```python
from build123d import *

# Parameters (mm, degrees)
SKETCH1_R           = 71.12
SKETCH1_R_2         = 12.704134002
SKETCH1_R_3         = 6.35
BOSS_EXTRUDE1_DEPTH = 3.175


with BuildPart() as part:
    # Sketch1 → Boss-Extrude1 (new body, symmetric)
    with BuildSketch(Plane(origin=(0, 0, 0), x_dir=(1, 0, 0), z_dir=(0, 1, 0))):
        Circle(SKETCH1_R)
        with Locations((-25.296602045, 14.605)):
            Circle(SKETCH1_R_2, mode=Mode.SUBTRACT)
        with Locations((-25.296602045, -14.605)):
            Circle(SKETCH1_R_2, mode=Mode.SUBTRACT)
        with Locations((0, -29.21)):
            Circle(SKETCH1_R_2, mode=Mode.SUBTRACT)
        with Locations((25.296602045, -14.605)):
            Circle(SKETCH1_R_2, mode=Mode.SUBTRACT)
        with Locations((25.296602045, 14.605)):
            Circle(SKETCH1_R_2, mode=Mode.SUBTRACT)
        with Locations((0, 29.21)):
            Circle(SKETCH1_R_2, mode=Mode.SUBTRACT)
        Circle(SKETCH1_R_3, mode=Mode.SUBTRACT)
    extrude(amount=BOSS_EXTRUDE1_DEPTH, both=True)


solid = part.part
```
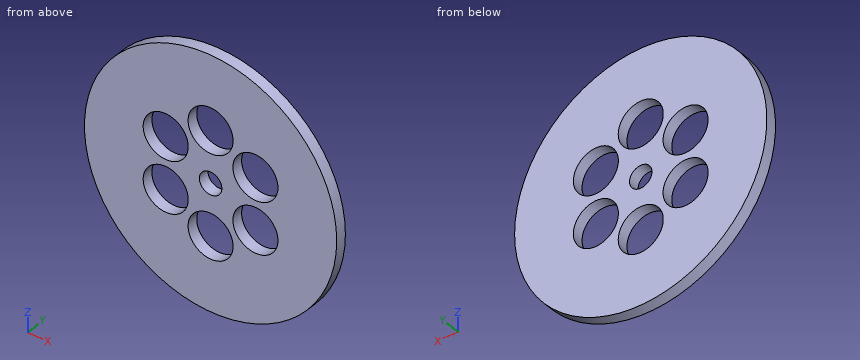
Geometry check sheet. Reference: the model listing, model coordinates, mm. Round coordinates to 2 decimals unless told otherwise and drop trailing zeros. Order: outer loops, then holes, each group sorted by start corner. A loop starts at its lowest first (then second) coordinate and runs counter-clockwise, first axis right, second up. Notation, with made-up numbers: (-21, 83) - (30, 83) arc R21 ccw to (30, 87) - close; hole circle Ø4 at (18, -17). An arc over 180 degrees is marked (long way). Use a Markdown table: item, result. Add a question column.
(1) Sectioned sample at D-D, the plane z = 0. Enter the section's corners in (x, y) (3 decimals).
(2) Sectioned sample at A-A, the plane x = 0. Enter the section's corners in (y, z) (3 decimals).
(3) Depth check by flat-ended pin: pin 1 (1.5 mm diameter, centred on y = -0.5, z = -31, fed in from +X); pin 2 (1.5 mm diameter, centred on y = 1.5, z = -30.5, fed in from -X). Enter the tip coordinate at first touch or a pass-through.
(4) Material ranges on line 1 along X through (y, z) = (1.5, 0); line 2 along Z through (x, y) = (-25.5, 1); line 3 along Z through (x, y) = (0, 0.5), recorded low to high. Write a range as [from, to].
(5) Sectioned sample at B-B, the plane z = 19. Enter the section's corners in (x, y) (3 decimals).
(6) Sectioned sample at C-C, the plane x = 21.5. Enter the section's corners in (y, z) (3 decimals), and give its area (3 significant figures).
Answers below:
| question | item | result |
|---|---|---|
| 1 | outline | (-71.12, -3.175) - (-6.35, -3.175) - (-6.35, 3.175) - (-71.12, 3.175) - close; (6.35, -3.175) - (71.12, -3.175) - (71.12, 3.175) - (6.35, 3.175) - close |
| 2 | outline | (-3.175, -71.12) - (3.175, -71.12) - (3.175, -41.914) - (-3.175, -41.914) - close; (-3.175, -16.506) - (3.175, -16.506) - (3.175, -6.35) - (-3.175, -6.35) - close; (-3.175, 6.35) - (3.175, 6.35) - (3.175, 16.506) - (-3.175, 16.506) - close; (-3.175, 41.914) - (3.175, 41.914) - (3.175, 71.12) - (-3.175, 71.12) - close |
| 3 | pin 1 | x = 64.37 |
| 3 | pin 2 | x = -64.6 |
| 4 | line 1 | [-71.12, -6.35], [6.35, 71.12] |
| 4 | line 2 | [-66.39, -27.31], [-1.9, 1.9], [27.31, 66.39] |
| 4 | line 3 | [-71.12, -41.91], [-16.51, -6.35], [6.35, 16.51], [41.91, 71.12] |
| 5 | outline | (-68.535, -3.175) - (-37.216, -3.175) - (-37.216, 3.175) - (-68.535, 3.175) - close; (-13.377, -3.175) - (-7.56, -3.175) - (-7.56, 3.175) - (-13.377, 3.175) - close; (7.56, -3.175) - (13.377, -3.175) - (13.377, 3.175) - (7.56, 3.175) - close; (37.216, -3.175) - (68.535, -3.175) - (68.535, 3.175) - (37.216, 3.175) - close |
| 6 | outline | (-3.175, -67.792) - (3.175, -67.792) - (3.175, -26.729) - (-3.175, -26.729) - close; (-3.175, -2.481) - (3.175, -2.481) - (3.175, 2.481) - (-3.175, 2.481) - close; (-3.175, 26.729) - (3.175, 26.729) - (3.175, 67.792) - (-3.175, 67.792) - close |
| 6 | area | 553 mm² |
